Part print with two shaded views. Sizes in mm from the minimum x, y, z corner. A direction names the side the tool comes from. Round coordinates to 2 decimals unless told otherwise and drop trailing zeros. Loops run counter-clockwise (first coordinate to the right, second up) from the corner with the lowest first, then second, coordinate; pieces in that order, holes last. Notation, with made-up numbers: (30.25, -28) -> (80.25, -28) arc R29 cw to (80.25, -4) -> close; hole circle Ø10 at (78.25, -0.75). An arc over 180 degrees is marked (long way). Answer as a JSON object with one key per item and string values. Group by question number.
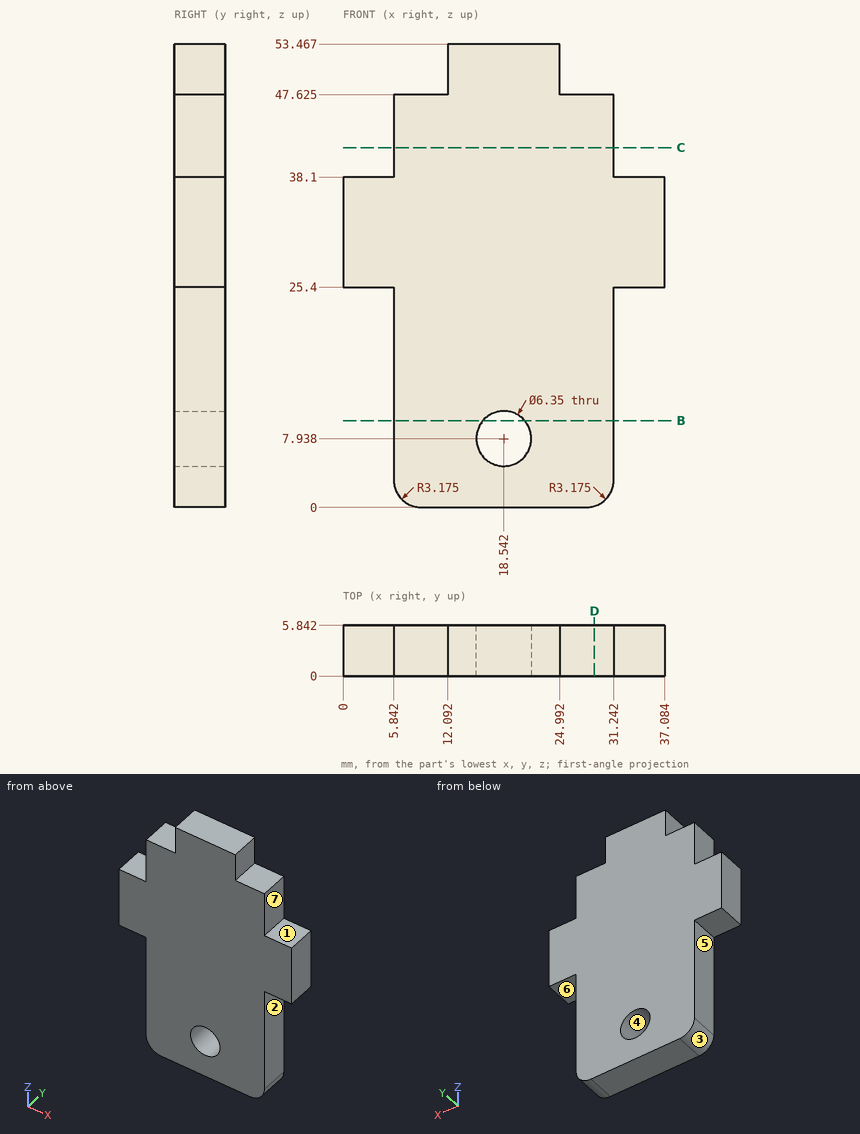
Item 1: Two-plate mould, pull along X, no slides. Class the marked faces 1, 2, 3 and 4: pulls with the +X half, pulls with the -X half, needs draft (parallel to the pull), parting line crosses it, or undercut.
Item 2: Band-saw the part on D-D, the plane x = 29. List the corners of the cut face in (y, z) (1 decimal).
Item 3: Band-saw the part on B-B, the plane z = 10. List the corners of the cut face in (x, y) (1 decimal).
Item 4: Drop flat-ended pins along their axis: pin 1 Ø3 at (y, z) = (1.5, 50) entering from +X; pin 2 Ø3 at (y, z) = (2, 41) entering from -X; pin 3 Ø3 at (x, y) = (4.5, 3.5) entering from +Z (1 decimal). Give the stop position or say it passes through.
Item 5: Drill centre lines: line 1 (X direction, y = 3.7, z = 51.5); line 2 (Z direction, x = 5, y = 2.75); line 3 (X direction, y = 4.8, z = 16.5). Where is each one in solid material? Low to high.
Item 6: Which spindle directions (+Z, -Z, +X, -X, +Y, -Y) get a long thin tool onto all of the face, cutting with end or side? Do the marked faces 5, 6 and 7. Say none if no direction does.
Item 7: Band-saw the part on C-C, the plane z = 41.5. List the corners of the cut face in (x, y).
Entries:
{
 "1": {"face 1": "needs draft", "face 2": "pulls with the +X half", "face 3": "pulls with the -X half", "face 4": "undercut"},
 "2": {"outline": "(0, 0.1) -> (5.8, 0.1) -> (5.8, 47.6) -> (0, 47.6) -> close"},
 "3": {"outline": "(5.8, 0) -> (16.1, 0) -> (16.1, 5.8) -> (5.8, 5.8) -> close; (21, 0) -> (31.2, 0) -> (31.2, 5.8) -> (21, 5.8) -> close"},
 "4": {"pin 1": "x = 24.99", "pin 2": "x = 5.84", "pin 3": "z = 47.6"},
 "5": {"line 1": "12.09 to 24.99", "line 2": "25.4 to 38.1", "line 3": "5.84 to 31.24"},
 "6": {"face 5": "-Z, -X, +Y, -Y", "face 6": "-Z, +X, +Y, -Y", "face 7": "+Z, +X, +Y, -Y"},
 "7": {"outline": "(5.84, 0) -> (31.24, 0) -> (31.24, 5.84) -> (5.84, 5.84) -> close"}
}
